from build123d import *

# Parameters (mm, degrees)
SKETCH_W        = 115
SKETCH_H        = 78
PAD_DEPTH       = 27
SKETCH001_W     = 105
SKETCH001_H     = 68
POCKET_DEPTH    = 21
POCKET005_DEPTH = 5
SKETCH015_W     = 6
SKETCH015_H     = 11
SKETCH015_W_2   = 8
PAD006_DEPTH    = 15.5
SKETCH012_W     = 3
SKETCH012_H     = 3
SKETCH012_W_2   = 10
SKETCH012_W_3   = 11
PAD007_DEPTH    = 24
SKETCH016_R     = 1.7
HOLE_DEPTH      = 11.5
HOLE_TIPS_R     = 1.7
SKETCH017_R     = 1.7
HOLE001_DEPTH   = 20
HOLE001_TIPS_R  = 1.7
SKETCH018_W     = 36
SKETCH018_H     = 36
PAD008_DEPTH    = 2
SKETCH025_R     = 1.7
POCKET010_DEPTH = 1
SKETCH028_W     = 88
SKETCH028_H     = 2
POCKET011_DEPTH = 115.001
CHAMFER_SIZE    = 0.75


with BuildPart() as part:
    # Sketch → Pad (new body)
    with BuildSketch(Plane.XY):
        with Locations((52.5, 32)):
            Rectangle(SKETCH_W, SKETCH_H)
    extrude(amount=PAD_DEPTH)

    # Sketch001 (on Face6 of Pad) → Pocket (cut)
    with BuildSketch(Plane.XY.offset(27)):
        with Locations((52.5, 32)):
            Rectangle(SKETCH001_W, SKETCH001_H)
    extrude(amount=-POCKET_DEPTH, mode=Mode.SUBTRACT)

    # Sketch014 → Pocket005 (cut)
    with BuildSketch(Plane.YZ.offset(110)):
        with BuildLine():
            ThreePointArc((56.25908, 12.405), (53, 24.475), (49.74092, 12.405))
            Line((49.74092, 12.405), (56.25908, 12.405))
        make_face()
        with BuildLine():
            ThreePointArc((12.746425, 15.2), (11, 21.3), (9.253575, 15.2))
            Line((12.746425, 15.2), (9.253575, 15.2))
        make_face()
        with BuildLine():
            ThreePointArc((26.65, 15.069556), (32, 11.9), (37.35, 15.069556))
            Line((37.35, 20.930444), (37.35, 15.069556))
            ThreePointArc((37.35, 20.930444), (32, 24.1), (26.65, 20.930444))
            Line((26.65, 20.930444), (26.65, 15.069556))
        make_face()
    extrude(amount=-POCKET005_DEPTH, mode=Mode.SUBTRACT)

    # Sketch015 → Pad006 (join)
    with BuildSketch(Plane.XY.offset(3)):
        with Locations((3, 60.5)):
            Rectangle(SKETCH015_W, SKETCH015_H)
        with Locations((78, 60.5)):
            Rectangle(SKETCH015_W_2, SKETCH015_H)
    extrude(amount=PAD006_DEPTH)

    # Sketch012 → Pad007 (join)
    with BuildSketch(Plane.XY.offset(3)):
        with Locations((1.5, 64.5)):
            Rectangle(SKETCH012_W, SKETCH012_H)
        with Locations((103.5, 64.5)):
            Rectangle(SKETCH012_W, SKETCH012_H)
        with Locations((1.5, -0.5)):
            Rectangle(SKETCH012_W, SKETCH012_H)
        with Locations((73, 64.5)):
            Rectangle(SKETCH012_W_2, SKETCH012_H)
        with Locations((32, -0.5)):
            Rectangle(SKETCH012_W_2, SKETCH012_H)
        with Locations((73, -0.5)):
            Rectangle(SKETCH012_W_2, SKETCH012_H)
        with Locations((32.5, 64.5)):
            Rectangle(SKETCH012_W_3, SKETCH012_H)
        with Locations((103.5, -0.5)):
            Rectangle(SKETCH012_W, SKETCH012_H)
    extrude(amount=PAD007_DEPTH)

    # Sketch016 → Hole (cut)
    with BuildSketch(Plane.XY.offset(18.5)):
        with Locations((3.25, 59)):
            Circle(SKETCH016_R)
        with Locations((77, 59)):
            Circle(SKETCH016_R)
    extrude(amount=-HOLE_DEPTH, mode=Mode.SUBTRACT)

    # Hole tips → Hole tip 1 section 0
    with BuildSketch(Plane.XY.offset(7), mode=Mode.PRIVATE) as hole_tip_1_s0:
        with Locations((3.25, 59)):
            Circle(HOLE_TIPS_R)
    loft([hole_tip_1_s0.sketch, Vertex(3.25, 59, 5.978537)], mode=Mode.SUBTRACT)

    # Hole tips → Hole tip 2 section 0
    with BuildSketch(Plane.XY.offset(7), mode=Mode.PRIVATE) as hole_tip_2_s0:
        with Locations((77, 59)):
            Circle(HOLE_TIPS_R)
    loft([hole_tip_2_s0.sketch, Vertex(77, 59, 5.978537)], mode=Mode.SUBTRACT)

    # Sketch017 (on Face2 of Hole) → Hole001 (cut)
    with BuildSketch(Plane.XY.offset(27)):
        with Locations((-1, 67)):
            Circle(SKETCH017_R)
        with Locations((-1, -3)):
            Circle(SKETCH017_R)
        with Locations((73, 67)):
            Circle(SKETCH017_R)
        with Locations((73, -3)):
            Circle(SKETCH017_R)
        with Locations((32, -3)):
            Circle(SKETCH017_R)
        with Locations((32, 67)):
            Circle(SKETCH017_R)
        with Locations((106, 67)):
            Circle(SKETCH017_R)
        with Locations((106, -3)):
            Circle(SKETCH017_R)
    extrude(amount=-HOLE001_DEPTH, mode=Mode.SUBTRACT)

    # Hole001 tips → Hole001 tip 1 section 0
    with BuildSketch(Plane.XY.offset(7), mode=Mode.PRIVATE) as hole001_tip_1_s0:
        with Locations((-1, 67)):
            Circle(HOLE001_TIPS_R)
    loft([hole001_tip_1_s0.sketch, Vertex(-1, 67, 5.978537)], mode=Mode.SUBTRACT)

    # Hole001 tips → Hole001 tip 2 section 0
    with BuildSketch(Plane.XY.offset(7), mode=Mode.PRIVATE) as hole001_tip_2_s0:
        with Locations((-1, -3)):
            Circle(HOLE001_TIPS_R)
    loft([hole001_tip_2_s0.sketch, Vertex(-1, -3, 5.978537)], mode=Mode.SUBTRACT)

    # Hole001 tips → Hole001 tip 3 section 0
    with BuildSketch(Plane.XY.offset(7), mode=Mode.PRIVATE) as hole001_tip_3_s0:
        with Locations((73, 67)):
            Circle(HOLE001_TIPS_R)
    loft([hole001_tip_3_s0.sketch, Vertex(73, 67, 5.978537)], mode=Mode.SUBTRACT)

    # Hole001 tips → Hole001 tip 4 section 0
    with BuildSketch(Plane.XY.offset(7), mode=Mode.PRIVATE) as hole001_tip_4_s0:
        with Locations((73, -3)):
            Circle(HOLE001_TIPS_R)
    loft([hole001_tip_4_s0.sketch, Vertex(73, -3, 5.978537)], mode=Mode.SUBTRACT)

    # Hole001 tips → Hole001 tip 5 section 0
    with BuildSketch(Plane.XY.offset(7), mode=Mode.PRIVATE) as hole001_tip_5_s0:
        with Locations((32, -3)):
            Circle(HOLE001_TIPS_R)
    loft([hole001_tip_5_s0.sketch, Vertex(32, -3, 5.978537)], mode=Mode.SUBTRACT)

    # Hole001 tips → Hole001 tip 6 section 0
    with BuildSketch(Plane.XY.offset(7), mode=Mode.PRIVATE) as hole001_tip_6_s0:
        with Locations((32, 67)):
            Circle(HOLE001_TIPS_R)
    loft([hole001_tip_6_s0.sketch, Vertex(32, 67, 5.978537)], mode=Mode.SUBTRACT)

    # Hole001 tips → Hole001 tip 7 section 0
    with BuildSketch(Plane.XY.offset(7), mode=Mode.PRIVATE) as hole001_tip_7_s0:
        with Locations((106, 67)):
            Circle(HOLE001_TIPS_R)
    loft([hole001_tip_7_s0.sketch, Vertex(106, 67, 5.978537)], mode=Mode.SUBTRACT)

    # Hole001 tips → Hole001 tip 8 section 0
    with BuildSketch(Plane.XY.offset(7), mode=Mode.PRIVATE) as hole001_tip_8_s0:
        with Locations((106, -3)):
            Circle(HOLE001_TIPS_R)
    loft([hole001_tip_8_s0.sketch, Vertex(106, -3, 5.978537)], mode=Mode.SUBTRACT)

    # Sketch018 → Pad008 (join)
    with BuildSketch(Plane.XY.offset(6)):
        with Locations((40, 23)):
            Rectangle(SKETCH018_W, SKETCH018_H)
    extrude(amount=PAD008_DEPTH)

    # Sketch025 → Pocket010 (cut)
    with BuildSketch(Plane.XY.offset(27)):
        with BuildLine():
            ThreePointArc((-1, 70), (-3.12132, 69.12132), (-4, 67))
            Line((-4, -3), (-4, 67))
            ThreePointArc((-4, -3), (-3.12132, -5.12132), (-1, -6))
            Line((-1, -6), (106, -6))
            ThreePointArc((106, -6), (108.12132, -5.12132), (109, -3))
            Line((109, 66.999984), (109, -3))
            ThreePointArc((109, 66.999984), (108.121326, 69.121315), (106, 70))
            Line((-1, 70), (106, 70))
        make_face()
        with Locations((32, 67)):
            Circle(SKETCH025_R, mode=Mode.SUBTRACT)
        with Locations((32, -3)):
            Circle(SKETCH025_R, mode=Mode.SUBTRACT)
        with Locations((106, -3)):
            Circle(SKETCH025_R, mode=Mode.SUBTRACT)
        with Locations((106, 67)):
            Circle(SKETCH025_R, mode=Mode.SUBTRACT)
        with BuildLine():
            Line((-2, 64.171573), (-2, -0.171573))
            ThreePointArc((1.828427, -4), (1.12132, -0.87868), (-2, -0.171573))
            Line((29.171573, -4), (1.828427, -4))
            ThreePointArc((34.828427, -4), (32, 0), (29.171573, -4))
            Line((70.171573, -4), (34.828427, -4))
            ThreePointArc((75.828427, -4), (73, 0), (70.171573, -4))
            Line((75.828427, -4), (103.171573, -4))
            ThreePointArc((107, -0.171573), (103.87868, -0.87868), (103.171573, -4))
            Line((107, 64.171573), (107, -0.171573))
            ThreePointArc((103.171573, 68), (103.87868, 64.87868), (107, 64.171573))
            Line((75.828427, 68), (103.171573, 68))
            ThreePointArc((70.171573, 68), (73, 64), (75.828427, 68))
            Line((34.828427, 68), (70.171573, 68))
            ThreePointArc((29.171573, 68), (32, 64), (34.828427, 68))
            Line((1.828427, 68), (29.171573, 68))
            ThreePointArc((-2, 64.171573), (1.12132, 64.87868), (1.828427, 68))
        make_face(mode=Mode.SUBTRACT)
    extrude(amount=-POCKET010_DEPTH, mode=Mode.SUBTRACT)

    # Sketch028 (on Face87 of Pocket010) → Pocket011 (cut, through all)
    with BuildSketch(Plane.YZ.offset(110)):
        with Locations((27, 1)):
            Rectangle(SKETCH028_W, SKETCH028_H)
    extrude(amount=-POCKET011_DEPTH, mode=Mode.SUBTRACT)

    # Chamfer
    chamfer_edges = [part.edges().sort_by_distance(p)[0] for p in [
        (52.5, -7, 2),
        (-5, -7, 14.5),
        (110, -7, 14.5),
        (110, 32, 2),
        (110, 71, 14.5),
        (52.5, 71, 2),
        (-5, 71, 14.5),
        (-5, 32, 2),
    ]]
    chamfer(chamfer_edges, length=CHAMFER_SIZE)


with BuildPart() as part_1:
    # Body placement: moved
    add(part.part.moved(Location((0, 0, -2.5))))


solid = part_1.part
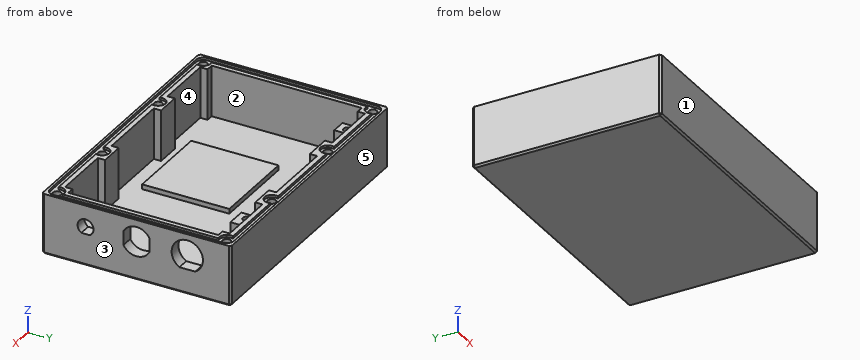
Model file for the job. Use its own axes, mm. Face numbers are marked on the shaded views. A direction names the side the tool comes from. Coordinates: 2 decimals unless noted, no trailing zeros. Order: outer loops, then holes, each group sorted by start corner. A loop starts at its lowest first (then second) coordinate and runs counter-clockwise, first axis right, second up. Notation, with made-up numbers: M -2,60.5 L 49,60.5 A20 ccw 49,94.5 Z; hole C 54.5,-14 d6. An arc over 180 degrees is marked long. Return JSON: item names as keys, results as strings.
1. Pull direction X, two halves, no side cores. Call the marked faces 1, 2 and 3: +X half, -X half, draft (parallel to the pull), parting line (faces both ways), or undercut.
Ans:
{"face 1": "draft", "face 2": "undercut", "face 3": "+X half"}
2. Saw through at A-A (y = 11). Give the cut face in (x, z), and give its area (3 significant figures).
Ans:
{"outline": "M -5,0.25 L -4.25,-0.5 L 109.25,-0.5 L 110,0.25 L 110,12.7 L 105,12.7 L 105,3.5 L 58,3.5 L 58,5.5 L 22,5.5 L 22,3.5 L 0,3.5 L 0,24.5 L -2,24.5 L -2,23.5 L -4,23.5 L -4,24.5 L -5,24.5 Z; M 105,18.8 L 110,18.8 L 110,24.5 L 109,24.5 L 109,23.5 L 107,23.5 L 107,24.5 L 105,24.5 Z", "area": "707 mm^2"}
3. Saw through at B-B (x = 41). Give the cut face in (y, z).
Ans:
{"outline": "M -7,0.25 L -6.25,-0.5 L 70.25,-0.5 L 71,0.25 L 71,24.5 L 70,24.5 L 70,23.5 L 68,23.5 L 68,24.5 L 66,24.5 L 66,3.5 L 41,3.5 L 41,5.5 L 5,5.5 L 5,3.5 L -2,3.5 L -2,24.5 L -4,24.5 L -4,23.5 L -6,23.5 L -6,24.5 L -7,24.5 Z"}
4. Saw through at C-C (y = 53). Give the cut face in (x, z) (3 decimals), and give its area (3 significant figures).
Ans:
{"outline": "M -5,0.25 L -4.25,-0.5 L 109.25,-0.5 L 110,0.25 L 110,9.905 L 105,9.905 L 105,3.5 L 0,3.5 L 0,24.5 L -2,24.5 L -2,23.5 L -4,23.5 L -4,24.5 L -5,24.5 Z; M 105,21.975 L 110,21.975 L 110,24.5 L 109,24.5 L 109,23.5 L 107,23.5 L 107,24.5 L 105,24.5 Z", "area": "605 mm^2"}
5. Tool access for the marked faces 4 and 5: list every direction of +Z, -Z, +X, -X, +Y, -Y with a clear straight run to the whole face (end or side of a thin tool).
Ans:
{"face 4": "+Z", "face 5": "+Z, -Z, +X, -X, +Y"}
6. Saw through at D-D (x = 80.5). Give the cut face in (y, z), and give its area (3 significant figures).
Ans:
{"outline": "M -7,0.25 L -6.25,-0.5 L 70.25,-0.5 L 71,0.25 L 71,24.5 L 70,24.5 L 70,23.5 L 68,23.5 L 68,24.5 L 66,24.5 L 66,16 L 55,16 L 55,3.5 L -2,3.5 L -2,24.5 L -4,24.5 L -4,23.5 L -6,23.5 L -6,24.5 L -7,24.5 Z", "area": "655 mm^2"}
7. Drill centre lines: probe 1 along Y at (x, z) = (73, 18); probe 2 along X at (y, z) = (64, 6.5); probe 3 along Y at (x, z) = (77, 9.25). Where is each one in solid material? Low to high.
Ans:
{"probe 1": "-7 to -4.7, -1.3 to 1, 63 to 65.3, 68.7 to 71", "probe 2": "-5 to 6, 27 to 38, 68 to 82, 102 to 110", "probe 3": "-7 to 1, 55 to 57.3, 60.7 to 71"}
8. Flat gauge pin, fed straight in: pin 1 (2.5 mm diameter, centred on x = 3.25, y = 59, fed in from +Z). Where does the tip first touch, or does it go through?
Ans:
{"pin 1": "z = 4.23"}
